Check sheet for the drawn part. Datum: minimum x, y, z corner. Units: mm. A direction names the side the tool comes from. Round coordinates to 2 decimals unless told otherwise and drop trailing zeros. Write each loop counter-clockwise with the first axis right and the second up, starting at its lowest first coordinate (ties: lowest second). Pieces come first, ordered by that corner, then holes.
Item 1: Go/stop test with flat-tipped pins: pin 1 Ø6 at (x, z) = (43.5, 73) entering from -Y; pin 2 Ø5.5 at (x, z) = (65.5, 11) entering from -Y (3 decimals); pin 3 Ø8 at (x, y) = (41, 8.5) entering from +Z; pin 4 Ø8 at (x, y) = (40, 4.5) entering from -Z. Record where each tip stops, or that it passes through.
Item 2: Release check for a two-part mould opening along Y. For the marked faces 1, 2 and 3 record: +Y half, -Y half, draft (parallel to the pull), parting line (faces both ways), or undercut.
Item 3: Material ranges on line 1 (X direction, y = 23, z = 50.5); line 2 (Z direction, x = 76.2, y = 7); line 3 (Z direction, x = 76.2, y = 19), recorded low to high.
Item 4: Tool access check on the marked faces 4 and 5. Record the directions out of +Z, -Z, +X, -X, +Y, -Y that give a thin tool (end or side, any length) a straight path to the whole face; none if there is none.
Item 5: Cross-section at A-A on z = 50.8. Enter the section's corners in (x, y), plus the area to 3 significant figures.
Item 6: Cross-section at D-D on x = 125. Enter the section's corners in (y, z) (3 decimals), plus the area to 3 significant figures.
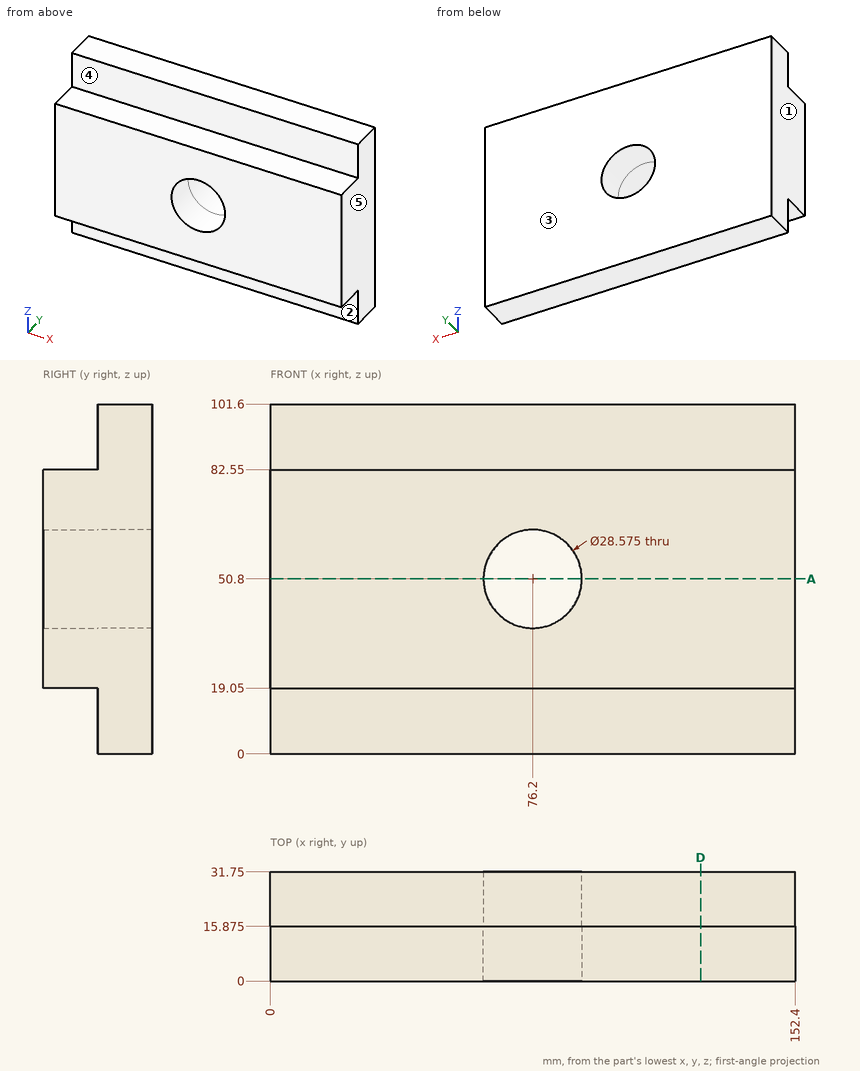
Response values:
1. pin 1: stops at y = 0
1. pin 2: stops at y = 15.875
1. pin 3: stops at z = 82.55
1. pin 4: stops at z = 19.05
2. face 1: draft
2. face 2: -Y half
2. face 3: +Y half
3. line 1: x = 0 to 61.92, 90.48 to 152.4
3. line 2: z = 19.05 to 36.51, 65.09 to 82.55
3. line 3: z = 0 to 36.51, 65.09 to 101.6
4. face 4: +Z, +X, -X, -Y
4. face 5: +Z, -Z, +X, +Y, -Y
5. outline: (0, 0) - (61.91, 0) - (61.91, 31.75) - (0, 31.75) - close; (90.49, 0) - (152.4, 0) - (152.4, 31.75) - (90.49, 31.75) - close
5. area: 3,930 mm2
6. outline: (0, 19.05) - (15.875, 19.05) - (15.875, 0) - (31.75, 0) - (31.75, 101.6) - (15.875, 101.6) - (15.875, 82.55) - (0, 82.55) - close
6. area: 2,620 mm2
